```python
from build123d import *

# Parameters (mm, degrees)
F1_DEPTH  = 10
F4_DEPTH  = 2
F7_R      = 2.6
F8_DEPTH  = 10
F9_DEPTH  = 10
F10_DEPTH = 2
F6_R      = 2.6
F11_DEPTH = 10


with BuildPart() as f1:
    # F0 (on Front) → F1 (new body, symmetric)
    with BuildSketch(Plane.XZ):
        Polygon((12.8, 8), (0, 8), (-12.8, 8), (-5, 0.2), (-5, 0), (0, 0), (5, 0), (5, 0.2), align=None)
    extrude(amount=F1_DEPTH, both=True)

    # F3 (on Front) → F4 (cut, symmetric)
    with BuildSketch(Plane.XZ):
        Polygon((2.3094010768, 0), (4.6188021535, 4), (4.6188021535, 8), (-4.6188021535, 8), (-4.6188021535, 4), (-2.3094010768, 0), align=None)
    extrude(amount=F4_DEPTH, both=True, mode=Mode.SUBTRACT)

    # F7 (on Front) → F8 (cut, symmetric)
    with BuildSketch(Plane.XZ):
        with Locations((0, 4)):
            Circle(F7_R)
    extrude(amount=F8_DEPTH, both=True, mode=Mode.SUBTRACT)

    # F2 (on Right) → F9 (join, symmetric)
    with BuildSketch(Plane.YZ):
        Polygon((-5, 0), (-5, -0.2), (-12.8, -8), (0, -8), (12.8, -8), (5, -0.2), (5, 0), (0, 0), align=None)
    extrude(amount=F9_DEPTH, both=True)

    # F5 (on Right) → F10 (cut, symmetric)
    with BuildSketch(Plane.YZ):
        Polygon((-2.3094010768, 0), (-4.6188021535, -4), (-4.6188021535, -8), (4.6188021535, -8), (4.6188021535, -4), (2.3094010768, 0), align=None)
    extrude(amount=F10_DEPTH, both=True, mode=Mode.SUBTRACT)

    # F6 (on Right) → F11 (cut, symmetric)
    with BuildSketch(Plane.YZ):
        with Locations((0, -4)):
            Circle(F6_R)
    extrude(amount=F11_DEPTH, both=True, mode=Mode.SUBTRACT)


solid = f1.part
```
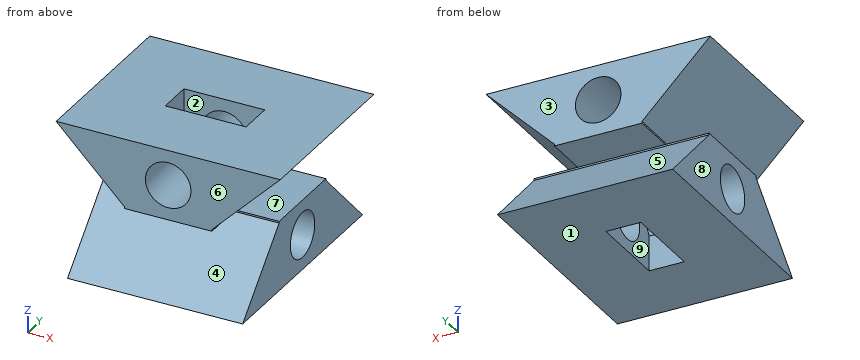
Design review of the part built by this model. Coordinates are the model's own, in mm. Face numbers are marked on the shaded views. A direction names the side the tool comes from. Coordinates: 2 decimals unless noted, no trailing zeros. Loops run counter-clockwise (first coordinate to the right, second up) from the corner with the lowest first, then second, coordinate; pieces in that order, holes last.
Q1. For pin 1 (1.2 mm diameter, centred on y = 0.5, z = 6, fed in from -X); pin 2 (8 mm diameter, centred on x = 7, z = 2, fed in from +Y); pin 3 (9 mm diameter, centred on y = 5, z = -3, fed in from -X); pin 4 (3 mm diameter, centred on y = 0, z = -4, fed in from -X), all flat-tipped, find the tip position at first contact; note any pin that passes through.
Reported:
pin 1: stops at x = -11.4
pin 2: stops at y = 10
pin 3: stops at x = -10
pin 4: passes through
Q2. We need section A-A on y = -6. State the section outline as (x, z) points.
Reported:
outline: (-12.8, 8) - (-5, 0.2) - (-5, 0) - (5, 0) - (5, 0.2) - (12.8, 8) - close; (-10, -8) - (10, -8) - (10, -1.2) - (-10, -1.2) - close; hole circle Ø5.2 at (0, 4)
Q3. We need section B-B on x = -9.25. State the section outline as (y, z) points.
Reported:
outline: (-12.8, -8) - (12.8, -8) - (5, -0.2) - (5, 0) - (-5, 0) - (-5, -0.2) - close; (-10, 4.45) - (10, 4.45) - (10, 8) - (-10, 8) - close; hole circle Ø5.2 at (0, -4)
Q4. Tool access review of the marked faces 5, 6, 7, 8 and 9: name each direction out of +Z, -Z, +X, -X, +Y, -Y from which nothing blocks a thin tool from reaching the whole face with its end or side.
Reported:
face 5: +X, -X, +Y
face 6: +Z, +X, -X, -Y
face 7: +X, +Y, -Y
face 8: -Z, -X, +Y, -Y
face 9: -Z
Q5. We need section C-C on x = 0. State the section outline as (y, z) points.
Reported:
outline: (-12.8, -8) - (-4.62, -8) - (-4.62, -4) - (-2.31, 0) - (-2, 0) - (-2, 1.4) - (-10, 1.4) - (-10, 0) - (-5, 0) - (-5, -0.2) - close; (-10, 6.6) - (-2, 6.6) - (-2, 8) - (-10, 8) - close; (2, 0) - (2.31, 0) - (4.62, -4) - (4.62, -8) - (12.8, -8) - (5, -0.2) - (5, 0) - (10, 0) - (10, 1.4) - (2, 1.4) - close; (2, 6.6) - (10, 6.6) - (10, 8) - (2, 8) - close
Q6. We need section D-D on y = 0. State the section outline as (x, z) points.
Reported:
outline: (-12.8, 8) - (-5, 0.2) - (-5, 0) - (-10, 0) - (-10, -1.4) - (-2, -1.4) - (-2, 0) - (-2.31, 0) - (-4.62, 4) - (-4.62, 8) - close; (-10, -8) - (-2, -8) - (-2, -6.6) - (-10, -6.6) - close; (2, -8) - (10, -8) - (10, -6.6) - (2, -6.6) - close; (2, -1.4) - (10, -1.4) - (10, 0) - (5, 0) - (5, 0.2) - (12.8, 8) - (4.62, 8) - (4.62, 4) - (2.31, 0) - (2, 0) - close
Q7. To check wall thickness, follow line 1 (Z direction, x = 9.5, y = 0.5); line 2 (Z direction, x = 0, y = 8); line 3 (X direction, y = 3, z = -0.25). State the ranges of each line that lie inside material, in increasing order.
Reported:
line 1: z = -8 to -6.55, -1.45 to 0, 4.7 to 8
line 2: z = -8 to -3.2, 0 to 1.4, 6.6 to 8
line 3: x = -10 to 10
Q8. The part is to be moulded in two halves that separate along Y. For the marked faces 1, 2, 3 and 4, say which applies: +Y half, -Y half, draft (parallel to the pull), parting line (faces both ways), or undercut.
Reported:
face 1: draft
face 2: undercut
face 3: +Y half
face 4: -Y half
